Model file for the job. Use its own axes, mm. Coordinates: 2 decimals unless noted, no trailing zeros. Write each loop counter-clockwise with the first axis right and the second up, starting at its lowest first coordinate (ties: lowest second). Pieces come first, ordered by that corner, then holes.
Q1. Drill centre lines: probe 1 along X at (y, z) = (-0.1, 81); probe 2 along Y at (x, z) = (-54.95, 45); probe 3 along Y at (x, z) = (-55.2, 74). Where is each one in solid material? Low to high.
Q2. Band-saw the part on A-A, the plane z = 69.5. Write the cut outline in (x, y), plus the area to 3 significant figures.
Q3. Pin check, flat tip, straight feed: P1, Ø3, axis at x = -53, z = 70.5, coming from the -Y side. Stop position of the tip, or through.
from build123d import *

# Parameters (mm, degrees)
RESSALTO_EXTRUS_O1_DEPTH = 95
FILETE1_R                = 0.5
ESBO_O2_R                = 0.701481341
CORTE_EXTRUS_O1_DEPTH    = 112.084775939


with BuildPart() as part:
    # Esboço1 → Ressalto-extrusão1 (new body)
    with BuildSketch(Plane.XY.offset(135)):
        Polygon((-55.002122675, 2.886751346), (-57.502122675, 1.443375673), (-57.502122675, -1.443375673), (-55.002122675, -2.886751346), (-52.502122675, -1.443375673), (-52.502122675, 1.443375673), align=None)
    extrude(amount=-RESSALTO_EXTRUS_O1_DEPTH)

    # Filete1
    filete1_edges = [part.edges().sort_by_distance(p)[0] for p in [
        (-57.502122675, 0, 40),
        (-56.252122675, -2.165063509, 40),
        (-53.752122675, -2.165063509, 40),
        (-52.502122675, 0, 40),
        (-53.752122675, 2.165063509, 40),
        (-52.502122675, 0, 135),
        (-53.752122675, -2.165063509, 135),
        (-56.252122675, -2.165063509, 135),
        (-57.502122675, 0, 135),
        (-56.252122675, 2.165063509, 135),
        (-53.752122675, 2.165063509, 135),
        (-56.252122675, 2.165063509, 40),
    ]]
    fillet(filete1_edges, radius=FILETE1_R)

    # Esboço2 → Corte-extrusão1 (cut, through all)
    with BuildSketch(Plane.XY.offset(135)):
        with Locations((-55.002122675, 0)):
            Circle(ESBO_O2_R)
    extrude(amount=-CORTE_EXTRUS_O1_DEPTH, mode=Mode.SUBTRACT)


solid = part.part
Answer sheet:
1. probe 1: x = -57.5 to -55.7, -54.31 to -52.5
1. probe 2: y = -2.86 to -0.7, 0.7 to 2.86
1. probe 3: y = -2.77 to -0.67, 0.67 to 2.77
2. outline: (-57.5, -1.44) - (-55, -2.89) - (-52.5, -1.44) - (-52.5, 1.44) - (-55, 2.89) - (-57.5, 1.44) - close; hole circle Ø1.4 at (-55, 0)
2. area: 20.1 mm2
3. P1: stops at y = -2.6
